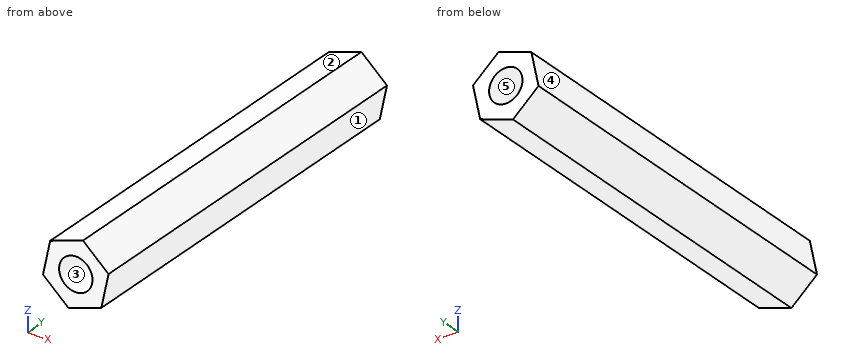
from build123d import *

# Parameters (mm, degrees)
RESSALTO_EXTRUS_O1_DEPTH                    = 37
FURO_ROSCADO_PARA_CONDU_TE_DE_M3X0_51_D     = 3.15
FURO_ROSCADO_PARA_CONDU_TE_DE_M3X0_51_DEPTH = 10
FURO_ROSCADO_PARA_CONDU_TE_DE_M3X0_51_TIP   = 0.946355475
FURO_ROSCADO_PARA_CONDU_TE_DE_M3X0_52_D     = 3.15
FURO_ROSCADO_PARA_CONDU_TE_DE_M3X0_52_DEPTH = 10
FURO_ROSCADO_PARA_CONDU_TE_DE_M3X0_52_TIP   = 0.946355475


with BuildPart() as part:
    # Esboço1 → Ressalto-extrusão1 (new body)
    with BuildSketch(Plane(origin=(0, 0, 0), x_dir=(1, 0, 0), z_dir=(0, 1, 0))):
        Polygon((3.092003015, -1.00100817), (2.412900012, 2.177249074), (-0.679103003, 3.178257244), (-3.092003015, 1.00100817), (-2.412900012, -2.177249074), (0.679103003, -3.178257244), align=None)
    extrude(amount=RESSALTO_EXTRUS_O1_DEPTH)

    # Furo roscado para conduíte de M3x0.51
    with Locations(Plane(origin=(0, 0, 0), x_dir=(-1, 0, 0), z_dir=(0, -1, 0))):
        with Locations((0, 0)):
            Hole(FURO_ROSCADO_PARA_CONDU_TE_DE_M3X0_51_D / 2, depth=FURO_ROSCADO_PARA_CONDU_TE_DE_M3X0_51_DEPTH)
            with Locations((0, 0, -(FURO_ROSCADO_PARA_CONDU_TE_DE_M3X0_51_DEPTH + FURO_ROSCADO_PARA_CONDU_TE_DE_M3X0_51_TIP / 2))):  # 118° drill point
                Cone(0, FURO_ROSCADO_PARA_CONDU_TE_DE_M3X0_51_D / 2, FURO_ROSCADO_PARA_CONDU_TE_DE_M3X0_51_TIP, mode=Mode.SUBTRACT)

    # Furo roscado para conduíte de M3x0.52
    with Locations(Plane(origin=(0, 37, 0), x_dir=(1, 0, 0), z_dir=(0, 1, 0))):
        with Locations((0, 0)):
            Hole(FURO_ROSCADO_PARA_CONDU_TE_DE_M3X0_52_D / 2, depth=FURO_ROSCADO_PARA_CONDU_TE_DE_M3X0_52_DEPTH)
            with Locations((0, 0, -(FURO_ROSCADO_PARA_CONDU_TE_DE_M3X0_52_DEPTH + FURO_ROSCADO_PARA_CONDU_TE_DE_M3X0_52_TIP / 2))):  # 118° drill point
                Cone(0, FURO_ROSCADO_PARA_CONDU_TE_DE_M3X0_52_D / 2, FURO_ROSCADO_PARA_CONDU_TE_DE_M3X0_52_TIP, mode=Mode.SUBTRACT)


solid = part.part
Geometry check sheet. Reference: the model listing, model coordinates, mm. Face numbers are marked on the shaded views. A direction names the side the tool comes from. Coordinates: 2 decimals unless noted, no trailing zeros. Order: outer loops, then holes, each group sorted by start corner. A loop starts at its lowest first (then second) coordinate and runs counter-clockwise, first axis right, second up. Notation, with made-up numbers: (80.25, 81.5) - (133.25, 81.5) arc R21 cw to (133.25, 85.5) - close; hole circle Ø11 at (-20, 69.5). An arc over 180 degrees is marked (long way). One line per item, written item: value.
(1) Thickness scan on probe 1 along X at (y, z) = (9, -0.5); probe 2 along Z at (x, y) = (0, 4.25) (3 decimals); probe 3 along Z at (x, y) = (0.25, 29.5). Record the ranges inside material, lowest first. Write a range as from..to.
Data:
probe 1: x = -2.98..-1.49, 1.49..2.77
probe 2: z = -2.958..-1.575, 1.575..2.958
probe 3: z = -2.88..-1.56, 1.56..3.04
(2) Depth check by flat-ended pin: pin 1 Ø3 at (x, z) = (0, 0) entering from -Y; pin 2 Ø2 at (y, z) = (11.5, 2.5) entering from -X; pin 3 Ø1 at (x, y) = (2, 4.5) entering from -Z. Enter the tip coordinate at first touch or a pass-through.
Data:
pin 1: stops at y = 10.05
pin 2: stops at x = -2.56
pin 3: stops at z = -2.47
(3) Release check for a two-part mould opening along X. For the marked faces 1, 2 and 3 record: +X half, -X half, draft (parallel to the pull), parting line (faces both ways), or undercut.
Data:
face 1: +X half
face 2: -X half
face 3: undercut
(4) Access from +Z, -Z, +X, -X, +Y, -Y to the whole of each face (thin tool, end or side, straight path). Record for the marked faces 4 and 5.
Data:
face 4: +Z, -X, +Y, -Y
face 5: +Y
(5) Sectioned sample at A-A (y = 20). Enter the section's corners in (x, z).
Data:
outline: (-3.09, -1) - (-0.68, -3.18) - (2.41, -2.18) - (3.09, 1) - (0.68, 3.18) - (-2.41, 2.18) - close
